from build123d import *

# Parameters (mm, degrees)
SKETCH_1_W          = 80
SKETCH_1_H          = 60
EXTRUDE_1_DEPTH     = 30
SKETCH_2_R          = 5
CUT_EXTRUDE_1_DEPTH = 61
SKETCH_3_W          = 80
SKETCH_3_H          = 6
CUT_EXTRUDE_2_DEPTH = 5


with BuildPart() as part:
    # 草图1 → 凸台-拉伸1 (new body)
    with BuildSketch(Plane(origin=(0, 0, 0), x_dir=(1, 0, 0), z_dir=(0, 1, 0))):
        Rectangle(SKETCH_1_W, SKETCH_1_H)
    extrude(amount=EXTRUDE_1_DEPTH)

    # 草图2 → 切除-拉伸1 (cut, through all)
    with BuildSketch(Plane.XY.offset(30)):
        with Locations((0, 15)):
            Circle(SKETCH_2_R)
    extrude(amount=-CUT_EXTRUDE_1_DEPTH, mode=Mode.SUBTRACT)

    # 草图3 → 切除-拉伸2 (cut)
    with BuildSketch(Plane(origin=(0, 30, 0), x_dir=(1, 0, 0), z_dir=(0, 1, 0))):
        with Locations((0, 15)):
            Rectangle(SKETCH_3_W, SKETCH_3_H)
        with Locations((0, -15)):
            Rectangle(SKETCH_3_W, SKETCH_3_H)
    extrude(amount=-CUT_EXTRUDE_2_DEPTH, mode=Mode.SUBTRACT)


solid = part.part
Geometry: final body of the model. Coordinates: model frame, mm. A direction names the side the tool comes from. Round coordinates to 2 decimals unless told otherwise and drop trailing zeros. Order: outer loops, then holes, each group sorted by start corner. A loop starts at its lowest first (then second) coordinate and runs counter-clockwise, first axis right, second up. Notation, with made-up numbers: (8.25, 4.25) - (44.25, 4.25) arc R15 cw to (44.25, 29.25) - close; hole circle Ø4 at (72.25, 85.5). An arc over 180 degrees is marked (long way). Write each question's results on one line, items separated by ' | '.
Item 1: Reachability of faces 1 (the flat face through (40, 15, 0)), 2 (the flat face through (-1, 28, 18)) from +Z, -Z, +X, -X, +Y, -Y: full face, straight path, thin tool, end or side. Return the list, or none.
Completed:
face 1: +Z, -Z, +X, +Y, -Y | face 2: +X, -X, +Y
Item 2: Section D-D, the plane y = 15. Return the cut outline in (x, z).
Completed:
outline: (-40, -30) - (-5, -30) - (-5, 30) - (-40, 30) - close; (5, -30) - (40, -30) - (40, 30) - (5, 30) - close
Item 3: Section A-A, the plane y = 19. Return the cut outline in (x, z), and give its area (3 significant figures).
Completed:
outline: (-40, -30) - (-3, -30) - (-3, 30) - (-40, 30) - close; (3, -30) - (40, -30) - (40, 30) - (3, 30) - close | area: 4,440 mm^2
Item 4: Material intervals for line 1 along Z through (x, y) = (-5, 26.75); line 2 along Y through (x, z) = (0, -15); line 3 along Y through (x, z) = (9, 16.5), sorted ascending. Write a range as [from, to].
Completed:
line 1: [-30, -18], [-12, 12], [18, 30] | line 2: [0, 10], [20, 25] | line 3: [0, 25]
Item 5: First-contact query: pin 1 Ø3 at (x, z) = (-11, -15.5) entering from +Y. Flat tip, straight axial feed; report the tip coordinate or a pass-through.
Completed:
pin 1: y = 25
Item 6: Section C-C, the plane z = -3.5. Return the cut outline in (x, y).
Completed:
outline: (-40, 0) - (40, 0) - (40, 30) - (-40, 30) - close; hole circle Ø10 at (0, 15)
Item 7: Section B-B, the plane x = 0. Return the cut outline in (y, z), and give its area (3 significant figures).
Completed:
outline: (0, -30) - (10, -30) - (10, 30) - (0, 30) - close; (20, -30) - (30, -30) - (30, -18) - (25, -18) - (25, -12) - (30, -12) - (30, 12) - (25, 12) - (25, 18) - (30, 18) - (30, 30) - (20, 30) - close | area: 1,140 mm^2
Item 8: Mould query, pull axis Z, two halves, no side actions, for faces 3 (the flat face through (-1, 8, 30)), 4 (the flat face through (-1, 30, 24)), 5 (the flat face through (-1, 25, 15)). Classes: pulls with the +Z half, pulls with the -Z half, needs draft (parallel to the pull), parting line crosses it, or undercut.
Completed:
face 3: pulls with the +Z half | face 4: needs draft | face 5: undercut
